Autodesk Inventor part; units mm, degrees
ref_plane "YZ Plane" through (0, 0, 0) normal (1, 0, 0) x (0, 1, 0)
ref_plane "XZ Plane" through (0, 0, 0) normal (0, 1, 0) x (-1, 0, 0)
ref_plane "XY Plane" through (0, 0, 0) normal (0, 0, 1) x (1, 0, 0)
sketch "Sketch1" plane through (0, 0, 0) normal (1, 0, 0) x (0, 1, 0)
  line L0 (31.4399, 11.0097) -> (31.4399, -9.3256)
  line L1 (31.4399, -9.3256) -> (49.0507, 0.842)
  line L2 (49.0507, 0.842) -> (31.4399, 11.0097)
  line L3 (46.6123, 0.842) -> (32.6591, -7.2139)
  line L4 (32.6591, -7.2139) -> (32.6591, 8.8979)
  line L5 (32.6591, 8.8979) -> (46.6123, 0.842)
  line L6 (49.0507, 0.842) -> (31.4399, -9.3256)
  line L7 (49.0507, -19.4932) -> (31.4399, -9.3256)
  line L8 (49.0507, 0.842) -> (49.0507, -19.4932)
  line L9 (47.8315, -1.2697) -> (33.8783, -9.3256)
  line L10 (33.8783, -9.3256) -> (47.8315, -17.3815)
  line L11 (47.8315, -17.3815) -> (47.8315, -1.2697)
  line L12 (31.4399, -9.3256) -> (31.4399, -29.6608)
  line L13 (31.4399, -29.6608) -> (49.0507, -19.4932)
  line L14 (32.6591, -27.5491) -> (32.6591, -11.4373)
  line L15 (32.6591, -11.4373) -> (46.6123, -19.4932)
  line L16 (46.6123, -19.4932) -> (32.6591, -27.5491)
  line L17 (49.0507, -19.4932) -> (49.0507, -39.8284)
  line L18 (49.0507, -39.8284) -> (31.4399, -29.6608)
  line L19 (47.8315, -37.7167) -> (47.8315, -21.6049)
  line L20 (33.8783, -29.6608) -> (47.8315, -37.7167)
  line L21 (47.8315, -21.6049) -> (33.8783, -29.6608)
  line L22 (31.4399, -29.6608) -> (31.4399, -49.9961)
  line L23 (32.6591, -47.8843) -> (32.6591, -31.7725)
  line L24 (31.4399, -49.9961) -> (49.0507, -39.8284)
  line L25 (46.6123, -39.8284) -> (32.6591, -47.8843)
  line L26 (32.6591, -31.7725) -> (46.6123, -39.8284)
  line L27 (49.0507, -39.8284) -> (49.0507, -60.1637)
  line L28 (47.8315, -41.9402) -> (33.8783, -49.9961)
  line L29 (33.8783, -49.9961) -> (47.8315, -58.052)
  line L30 (49.0507, -60.1637) -> (31.4399, -49.9961)
  line L31 (47.8315, -58.052) -> (47.8315, -41.9402)
  line L32 (31.4399, -49.9961) -> (31.4399, -70.3313)
  line L33 (31.4399, -70.3313) -> (49.0507, -60.1637)
  line L34 (46.6123, -60.1637) -> (32.6591, -68.2196)
  line L35 (32.6591, -68.2196) -> (32.6591, -52.1078)
  line L36 (32.6591, -52.1078) -> (46.6123, -60.1637)
  line L37 (31.4399, -9.3256) -> (13.8291, 0.842)
  line L38 (13.8291, 0.842) -> (31.4399, 11.0097)
  line L39 (16.2675, 0.842) -> (30.2207, -7.2139)
  line L40 (30.2207, -7.2139) -> (30.2207, 8.8979)
  line L41 (30.2207, 8.8979) -> (16.2675, 0.842)
  line L42 (31.4399, -9.3256) -> (13.8291, 0.842)
  line L43 (13.8291, -19.4932) -> (31.4399, -9.3256)
  line L44 (13.8291, 0.842) -> (13.8291, -19.4932)
  line L45 (15.0483, -1.2697) -> (29.0015, -9.3256)
  line L46 (29.0015, -9.3256) -> (15.0483, -17.3815)
  line L47 (15.0483, -17.3815) -> (15.0483, -1.2697)
  line L48 (13.8291, -19.4932) -> (31.4399, -9.3256)
  line L49 (31.4399, -29.6608) -> (13.8291, -19.4932)
  line L50 (30.2207, -11.4373) -> (16.2675, -19.4932)
  line L51 (30.2207, -27.5491) -> (30.2207, -11.4373)
  line L52 (16.2675, -19.4932) -> (30.2207, -27.5491)
  line L53 (13.8291, -39.8284) -> (31.4399, -29.6608)
  line L54 (16.2675, -39.8284) -> (30.2207, -47.8843)
  line L55 (30.2207, -47.8843) -> (30.2207, -31.7725)
  line L56 (31.4399, -49.9961) -> (13.8291, -39.8284)
  line L57 (30.2207, -31.7725) -> (16.2675, -39.8284)
  line L58 (31.4399, -29.6608) -> (13.8291, -19.4932)
  line L59 (15.0483, -21.6049) -> (29.0015, -29.6608)
  line L60 (13.8291, -19.4932) -> (13.8291, -39.8284)
  line L61 (15.0483, -37.7167) -> (15.0483, -21.6049)
  line L62 (13.8291, -39.8284) -> (31.4399, -29.6608)
  line L63 (29.0015, -29.6608) -> (15.0483, -37.7167)
  line L64 (13.8291, -60.1637) -> (31.4399, -49.9961)
  line L65 (30.2207, -68.2196) -> (30.2207, -52.1078)
  line L66 (31.4399, -70.3313) -> (13.8291, -60.1637)
  line L67 (30.2207, -52.1078) -> (16.2675, -60.1637)
  line L68 (16.2675, -60.1637) -> (30.2207, -68.2196)
  line L69 (31.4399, -49.9961) -> (13.8291, -39.8284)
  line L70 (13.8291, -39.8284) -> (13.8291, -60.1637)
  line L71 (15.0483, -58.052) -> (15.0483, -41.9402)
  line L72 (15.0483, -41.9402) -> (29.0015, -49.9961)
  line L73 (13.8291, -60.1637) -> (31.4399, -49.9961)
  line L74 (29.0015, -49.9961) -> (15.0483, -58.052)
  line L75 (13.8291, 0.842) -> (13.8291, 21.1773)
  line L76 (13.8291, 21.1773) -> (31.4399, 11.0097)
  line L77 (49.0507, 0.842) -> (49.0507, 21.1773)
  line L78 (49.0507, 21.1773) -> (31.4399, 11.0097)
  line L79 (49.0507, 21.1773) -> (13.8291, 21.1773)
  line L80 (49.0507, -60.1637) -> (49.0507, -80.4989)
  line L81 (49.0507, -80.4989) -> (31.4399, -70.3313)
  line L82 (13.8291, -60.1637) -> (13.8291, -80.4989)
  line L83 (13.8291, -80.4989) -> (31.4399, -70.3313)
  line L84 (49.0507, -80.4989) -> (13.8291, -80.4989)
  line L85 (15.0483, 2.9538) -> (15.0483, 19.0656)
  line L86 (29.0015, 11.0097) -> (15.0483, 2.9538)
  line L87 (15.0483, 19.0656) -> (29.0015, 11.0097)
  line L88 (47.8315, 2.9538) -> (47.8315, 19.0656)
  line L89 (47.8315, 19.0656) -> (33.8783, 11.0097)
  line L90 (33.8783, 11.0097) -> (47.8315, 2.9538)
  line L91 (33.8783, -70.3313) -> (47.8315, -78.3872)
  line L92 (47.8315, -78.3872) -> (47.8315, -62.2754)
  line L93 (47.8315, -62.2754) -> (33.8783, -70.3313)
  line L94 (29.0015, -70.3313) -> (15.0483, -78.3872)
  line L95 (15.0483, -78.3872) -> (15.0483, -62.2754)
  line L96 (15.0483, -62.2754) -> (29.0015, -70.3313)
  line L97 (33.4035, 19.9572) -> (43.2391, 19.9572)
  line L98 (43.2391, 19.9572) -> (31.4399, 12.4185)
  line L99 (31.4399, 12.4185) -> (18.3826, 19.9572)
  line L100 (18.3826, 19.9572) -> (33.4035, 19.9572)
  line L101 (33.4035, -79.2788) -> (43.2391, -79.2788)
  line L102 (43.2391, -79.2788) -> (31.4399, -71.7402)
  line L103 (31.4399, -71.7402) -> (18.3826, -79.2788)
  line L104 (18.3826, -79.2788) -> (33.4035, -79.2788)
  dimension "d13" = 1.2192
extrude "Extrusion1" add sketch "Sketch1" along normal blind 10
sketch "Sketch2" plane through (0, 13.8291, 21.1773) normal (0, 0, 1) x (1, 0, 0)
  line L0 (0, 35.2217) -> (10, 35.2217)
  circle A0 centre (5.0038, 17.6108) radius 1.27
  point P0 (0, -13.8291)
  point P1 (0, 17.6108)
extrude "Extrusion2" add sketch "Sketch2" along normal blind 3
sketch "Sketch3" plane through (0, 13.8291, -80.4989) normal (0, 0, -1) x (-1, 0, 0)
  line L0 (0, 35.2217) -> (-10, 35.2217)
  line L1 (0, 18.83) -> (-10, 18.83)
  circle A0 centre (-5, 18.83) radius 1.27
  point P0 (0, -13.8291)
  dimension "d36" = 2.54
extrude "Extrusion3" add sketch "Sketch3" along normal blind 3
properties part number "Arm support for bottom arms"
Work out the finished part from the listing and answer in its coordinate system (mm). Coordinates: 2 decimals unless noted, no trailing zeros. Loops run counter-clockwise (first coordinate to the right, second up) from the corner with the lowest first, then second, coordinate; pieces in that order, holes last. Notation, with made-up numbers: M -10.5,-9.75 L 27.5,-9.75 A18 ccw 27.5,10.25 Z; hole C 13.25,-38.75 d9. An arc over 180 degrees is marked long. Answer in a Markdown table with one row per item. Add a question column.
1. Find section B-B, the plane x = 9. State how many separate pieces and enclosed holes the cut face has, then the cut area to 3 significant figures.
2. Find section A-A, the plane z = -26. Write down the section's boundary in (x, y).
3. The mould has two halves that part along Y. Classify faces 1 (the flat face through (5, 49.051, -30)), 2 (the flat face through (6.04, 31.69, -80.499)), 3 (the flat face through (4.93, 40.95, -66.25)): pulls with the +Y half, pulls with the -Y half, needs draft (parallel to the pull), parting line crosses it, or undercut.
4. Flat-ended cylindrical pins translate along their axes: P1, Ø6, axis at x = 3, y = 43, coming from the -Z side; P2, Ø5, axis at x = 5, y = 26.5, coming from the +Z side. Find the tip coordinate at first contact, or state that the pin passes through.
5. Consider L1, parallel to Y at x = 6.5, z = -72; L2, parallel to Y at x = 2.5, z = 16.5; L3, parallel to Y at x = 4, z = -31.5. Determine where each line is inside the solid, lowest interval first.
Reported:
| question | item | result |
|---|---|---|
| 1 | separate pieces | 1 |
| 1 | enclosed holes | 20 |
| 1 | area | 1,370 mm^2 |
| 2 | outline | M 0,13.83 L 10,13.83 L 10,15.05 L 0,15.05 Z; M 0,22.66 L 10,22.66 L 10,27.54 L 0,27.54 Z; M 0,30.22 L 10,30.22 L 10,32.66 L 0,32.66 Z; M 0,35.34 L 10,35.34 L 10,40.22 L 0,40.22 Z; M 0,47.83 L 10,47.83 L 10,49.05 L 0,49.05 Z |
| 3 | face 1 | pulls with the +Y half |
| 3 | face 2 | needs draft |
| 3 | face 3 | undercut |
| 4 | P1 | stops at z = -80.5 |
| 4 | P2 | stops at z = 21.18 |
| 5 | L1 | y = 13.83 to 15.05, 26.11 to 30.99, 31.85 to 36.77, 47.83 to 49.05 |
| 5 | L2 | y = 13.83 to 15.05, 19.49 to 24.37, 37.83 to 43.39, 47.83 to 49.05 |
| 5 | L3 | y = 13.83 to 15.05, 25.82 to 37.06, 47.83 to 49.05 |
